Geometry: final body of the model. Coordinates: model frame, mm. A direction names the side the tool comes from. Coordinates: 2 decimals unless noted, no trailing zeros. Order: outer loops, then holes, each group sorted by start corner. A loop starts at its lowest first (then second) coordinate and runs counter-clockwise, first axis right, second up. Notation, with made-up numbers: M 81.25,-35.75 L 116.25,-35.75 A21 ccw 116.25,-0.75 Z; hole C -25,13.5 d5. An arc over 180 degrees is marked long. Write item = value, one per line.
from build123d import *

# Parameters (mm, degrees)
F0_R     = 12.5
F1_DEPTH = 4
F2_R     = 10.5
F3_DEPTH = 14
F4_R     = 5.734203
F5_DEPTH = 14


with BuildPart() as f1:
    # F0 (on Top) → F1 (new body)
    with BuildSketch(Plane.XY):
        Circle(F0_R)
    extrude(amount=F1_DEPTH)

    # F2 (on face) → F3 (join)
    with BuildSketch(Plane.XY.offset(4)):
        Circle(F2_R)
    extrude(amount=F3_DEPTH)

    # F4 (on face) → F5 (cut)
    with BuildSketch(Plane.XY.offset(4)):
        with Locations((-4.499399, 5.053002)):
            Circle(F4_R)
    extrude(amount=F5_DEPTH, mode=Mode.SUBTRACT)


solid = f1.part
1) Mould query, pull axis X, two halves, no side actions, for faces 1 (the face through (11.923, 3.755, 1.972)), 2 (the face through (0, 3, 4)), 3 (the face through (2, -2, 18)). Classes: pulls with the +X half, pulls with the -X half, needs draft (parallel to the pull), parting line crosses it, or undercut.
Numbers:
face_1 = parting line crosses it
face_2 = undercut
face_3 = needs draft
2) Set-up query: faces 4 (the face through (0, 0, 0)), 5 (the face through (6.69, -8.092, 10.902)). Return all of +Z, -Z, +X, -X, +Y, -Y with unobstructed straight access to the full face (end or side cutting, diameter ignored); none if empty.
Numbers:
face_4 = -Z, +X, -X, +Y, -Y
face_5 = +Z
3) Pin query (flat end, axial travel): pin 1 (1.5 mm diameter, centred on x = 8, z = 7.5, fed in from +Y); pin 2 (2 mm diameter, centred on y = 4.5, z = 12, fed in from +X); pin 3 (5 mm diameter, centred on x = 7.5, z = 4.5, fed in from -Y). Return the tip coordinate at first contact, or that it passes through.
Numbers:
pin_1 = 7.6
pin_2 = 9.9
pin_3 = -11.43
4) Section D-D, the plane x = 0.5. Return loops of the section in (y, z).
Numbers:
outline = M -12.49,0 L 12.49,0 L 12.49,4 L 10.49,4 L 10.49,18 L 7.86,18 L 7.86,4 L 2.24,4 L 2.24,18 L -10.49,18 L -10.49,4 L -12.49,4 Z
5) Section C-C, the plane z = 8.5. Return loops of the section in (x, y).
Numbers:
outline = M -9.96,3.31 A10.5 ccw long -2.14,10.28 A5.73 cw long Z
6) Line query: L1, parallel to X at y = 0.5, z = 15; L2, parallel to Y at x = -1.5, z = 14.75; L3, parallel to Z at x = -6.5, y = 7.75. Output: solid intervals per line, ascending.
Numbers:
L1 = -10.49 to -7.99, -1.01 to 10.49
L2 = -10.39 to 0.17, 9.94 to 10.39
L3 = 0 to 4
7) Section A-A, the plane x = -8.5. Return loops of the section in (y, z), and give its area (3 significant figures).
Numbers:
outline = M -9.17,0 L 9.17,0 L 9.17,4 L 0.94,4 L 0.94,18 L -6.16,18 L -6.16,4 L -9.17,4 Z
area = 173 mm²
8) Section B-B, the plane y = 5.5. Return loops of the section in (x, z).
Numbers:
outline = M -11.22,0 L 11.22,0 L 11.22,4 L 8.94,4 L 8.94,18 L 1.22,18 L 1.22,4 L -11.22,4 Z
